```python
from build123d import *

# Parameters (mm, degrees)
SKETCH1_R           = 1.5
SKETCH1_R_2         = 4.25
SKETCH1_R_3         = 5
SKETCH1_R_4         = 1
BOSS_EXTRUDE2_DEPTH = 5
SKETCH2_W           = 0.5
SKETCH2_H           = 37
BOSS_EXTRUDE3_DEPTH = 5
CUT_EXTRUDE1_DEPTH  = 10
BOSS_EXTRUDE4_DEPTH = 5
SKETCH5_R           = 1.6
CUT_EXTRUDE2_DEPTH  = 10
BOSS_EXTRUDE5_DEPTH = 5
SKETCH7_R           = 1
BOSS_EXTRUDE6_DEPTH = 5
SKETCH8_W           = 5
SKETCH8_H           = 37
CUT_EXTRUDE3_DEPTH  = 33


with BuildPart() as part:
    # Sketch1 → Boss-Extrude2 (new body)
    with BuildSketch(Plane.XY):
        with BuildLine():
            Line((45.25091594, -25.207708346), (50.00091594, -20.457708346))
            Line((50.00091594, -20.457708346), (50.00091594, 24.688738263))
            Line((50.00091594, 24.688738263), (45.147362549, 29.542291654))
            Line((45.147362549, 29.542291654), (26.35446933, 29.542291654))
            Line((26.35446933, 29.542291654), (21.25091594, 24.438738263))
            Line((21.25091594, 24.438738263), (21.25091594, 18.042291654))
            Line((21.25091594, 18.042291654), (20.408095363, 18.042291654))
            Line((20.408095363, 18.042291654), (16.70086026, 18.042291654))
            ThreePointArc((16.70086026, 18.042291654), (12.892426636, 17.542145454), (9.3422674, 16.075624987))
            ThreePointArc((9.3422674, 16.075624987), (2.182128173, 13.100539865), (-5.49908406, 12.043324729))
            Line((-5.49908406, 12.043324729), (-5.49908406, 12.039085999))
            ThreePointArc((-5.49908406, 12.039085999), (-15.49908406, 2.292291654), (-5.49908406, -7.454502691))
            Line((-5.49908406, -7.454502691), (-5.49908406, -7.458741422))
            ThreePointArc((-5.49908406, -7.458741422), (2.182128173, -8.515956557), (9.3422674, -11.491041679))
            ThreePointArc((9.3422674, -11.491041679), (12.892426636, -12.957562146), (16.70086026, -13.457708346))
            Line((16.70086026, -13.457708346), (20.408095363, -13.457708346))
            Line((20.408095363, -13.457708346), (21.25091594, -13.457708346))
            Line((21.25091594, -13.457708346), (21.25091594, -20.207708346))
            Line((21.25091594, -20.207708346), (26.25091594, -25.207708346))
            Line((26.25091594, -25.207708346), (45.25091594, -25.207708346))
        make_face()
        with Locations((46.75091594, -7.707708346)):
            Circle(SKETCH1_R, mode=Mode.SUBTRACT)
        with Locations((46.75091594, 12.292291654)):
            Circle(SKETCH1_R, mode=Mode.SUBTRACT)
        with Locations((33.50091594, 14.792291654)):
            Circle(SKETCH1_R_2, mode=Mode.SUBTRACT)
        with Locations((33.50091594, -10.207708346)):
            Circle(SKETCH1_R_2, mode=Mode.SUBTRACT)
        with Locations((19.25091594, 12.292291654)):
            Circle(SKETCH1_R, mode=Mode.SUBTRACT)
        with Locations((19.25091594, -7.707708346)):
            Circle(SKETCH1_R, mode=Mode.SUBTRACT)
        with Locations((-5.74908406, 2.292291654)):
            Circle(SKETCH1_R_3, mode=Mode.SUBTRACT)
        with Locations((1.25091594, 2.354746229)):
            Circle(SKETCH1_R_4, mode=Mode.SUBTRACT)
        with Locations((-5.686629485, -4.707708346)):
            Circle(SKETCH1_R_4, mode=Mode.SUBTRACT)
        with Locations((-12.74908406, 2.229837079)):
            Circle(SKETCH1_R_4, mode=Mode.SUBTRACT)
        with Locations((-5.811538636, 9.292291654)):
            Circle(SKETCH1_R_4, mode=Mode.SUBTRACT)
    extrude(amount=BOSS_EXTRUDE2_DEPTH)

    # Sketch2 → Boss-Extrude3 (add)
    with BuildSketch(Plane(origin=(0, 0, 0), x_dir=(-1, 0, 0), z_dir=(0, 0, -1))):
        Polygon((-26.25091594, -25.207708346), (-21.50091594, -25.207708346), (-21.50091594, -20.457708346), align=None)
        Polygon((-45.25091594, -25.207708346), (-45.50091594, -25.207708346), (-45.50091594, -24.957708346), align=None)
        Polygon((-45.50091594, 29.188738263), (-45.50091594, 29.792291654), (-21.50091594, 29.792291654), (-21.50091594, 24.688738263), (-26.35446933, 29.542291654), (-45.147362549, 29.542291654), align=None)
        with Locations((-50.25091594, 2.292291654)):
            Rectangle(SKETCH2_W, SKETCH2_H)
    extrude(amount=-BOSS_EXTRUDE3_DEPTH)

    # Sketch3 → Cut-Extrude1 (cut)
    with BuildSketch(Plane(origin=(0, 0, 0), x_dir=(-1, 0, 0), z_dir=(0, 0, -1))):
        Polygon((-50.00091594, -16.207708346), (-45.50091594, -16.207708346), (-45.50091594, -25.207708346), (-50.00091594, -20.457708346), align=None)
        Polygon((-50.50091594, 20.792291654), (-45.50091594, 20.792291654), (-45.50091594, 29.188738263), (-50.00091594, 24.688738263), align=None)
        Polygon((-21.50091594, -16.207708346), (-21.50091594, -20.457708346), (-21.25091594, -20.207708346), (-21.25091594, -16.207708346), align=None)
        Polygon((-21.50091594, 20.792291654), (-21.25091594, 20.792291654), (-21.25091594, 24.438738263), (-21.50091594, 24.688738263), align=None)
    extrude(amount=-CUT_EXTRUDE1_DEPTH, mode=Mode.SUBTRACT)

    # Sketch4 → Boss-Extrude4 (add)
    with BuildSketch(Plane(origin=(0, 0, 0), x_dir=(-1, 0, 0), z_dir=(0, 0, -1))):
        with BuildLine():
            Line((-21.25091594, 20.792291654), (-16.50091594, 20.792291654))
            Line((-16.50091594, 20.792291654), (-16.50091594, 18.040936414))
            ThreePointArc((-16.50091594, 18.040936414), (-16.600885803, 18.04195284), (-16.70086026, 18.042291654))
            Line((-16.70086026, 18.042291654), (-21.25091594, 18.042291654))
            Line((-21.25091594, 18.042291654), (-21.25091594, 20.792291654))
        make_face()
        with BuildLine():
            Line((-16.50091594, -13.456353106), (-16.50091594, -16.207708346))
            Line((-16.50091594, -16.207708346), (-21.25091594, -16.207708346))
            Line((-21.25091594, -16.207708346), (-21.25091594, -13.457708346))
            Line((-21.25091594, -13.457708346), (-16.70086026, -13.457708346))
            ThreePointArc((-16.70086026, -13.457708346), (-16.600885803, -13.457369532), (-16.50091594, -13.456353106))
        make_face()
    extrude(amount=-BOSS_EXTRUDE4_DEPTH)

    # Sketch5 → Cut-Extrude2 (cut)
    with BuildSketch(Plane.XY.offset(5)):
        with Locations((20.50091594, -7.707708346)):
            Circle(SKETCH5_R)
        with Locations((20.50091594, 12.292291654)):
            Circle(SKETCH5_R)
    extrude(amount=-CUT_EXTRUDE2_DEPTH, mode=Mode.SUBTRACT)

    # Sketch6 → Boss-Extrude5 (add)
    with BuildSketch(Plane.XY.offset(5)):
        with BuildLine():
            ThreePointArc((19.75191594, -6.293848735), (18.90091594, -7.707708346), (19.75191594, -9.121567957))
            ThreePointArc((19.75191594, -9.121567957), (17.75091594, -7.707708346), (19.75191594, -6.293848735))
        make_face()
        with BuildLine():
            ThreePointArc((19.75191594, 13.706151265), (18.90091594, 12.292291654), (19.75191594, 10.878432043))
            ThreePointArc((19.75191594, 10.878432043), (17.75091594, 12.292291654), (19.75191594, 13.706151265))
        make_face()
    extrude(amount=-BOSS_EXTRUDE5_DEPTH)

    # Sketch7 → Boss-Extrude6 (add)
    with BuildSketch(Plane(origin=(0, 0, 0), x_dir=(-1, 0, 0), z_dir=(0, 0, -1))):
        with Locations((-1.25091594, 2.354746229)):
            Circle(SKETCH7_R)
        with Locations((12.74908406, 2.229837079)):
            Circle(SKETCH7_R)
    extrude(amount=-BOSS_EXTRUDE6_DEPTH)

    # Sketch8 → Cut-Extrude3 (cut, through all)
    with BuildSketch(Plane.ZY.offset(-16.50091594)):
        with Locations((2.5, 2.292291654)):
            Rectangle(SKETCH8_W, SKETCH8_H)
    extrude(amount=CUT_EXTRUDE3_DEPTH, mode=Mode.SUBTRACT)


solid = part.part
```
The model under review builds one solid part; all positions refer to its coordinate system, in mm. A direction names the side the tool comes from. Round coordinates to 2 decimals unless told otherwise and drop trailing zeros. Order: outer loops, then holes, each group sorted by start corner. A loop starts at its lowest first (then second) coordinate and runs counter-clockwise, first axis right, second up.
(1) Take a section at C-C, the plane y = 22.5. State the section outline as (x, z) points.
Working result:
outline: (21.5, 0) - (45.5, 0) - (45.5, 5) - (21.5, 5) - close
(2) For P1, Ø2.5, axis at y = -21, z = 3, coming from the +X side; P2, Ø3, axis at x = 20.5, y = -7.71, coming from the +Z side; P3, Ø4, axis at x = 46.75, y = -7.71, coming from the -Z side; P4, Ø1.5, axis at y = 24.5, z = 1.5, coming from the -X side, all flat-tipped, find the tip position at first contact; note any pin that passes through.
Working result:
P1: stops at x = 45.5
P2: passes through
P3: stops at z = 0
P4: stops at x = 21.5
(3) Mouldability with a two-part tool opening along Y and no side actions: class faces 5 (the face through (21.501, -21, 2)), 6 (the face through (19, 20.792, 2)), 7 (the face through (30.4, 17.7, 2.5)) as released by +Y, released by -Y, zero draft, split by the parting line, or undercut.
Working result:
face 5: zero draft
face 6: released by +Y
face 7: undercut
(4) Take a section at B-B, the plane z = 4.1. State the section outline as (x, y) points, plus the area to 3 significant figures.
Working result:
outline: (16.5, -16.21) - (21.5, -16.21) - (21.5, -25.21) - (45.5, -25.21) - (45.5, -16.21) - (50.5, -16.21) - (50.5, 20.79) - (45.5, 20.79) - (45.5, 29.79) - (21.5, 29.79) - (21.5, 20.79) - (16.5, 20.79) - close; hole circle Ø3.2 at (20.5, -7.71); hole circle Ø3.2 at (20.5, 12.29); hole circle Ø8.5 at (33.5, -10.21); hole circle Ø8.5 at (33.5, 14.79); hole circle Ø3 at (46.75, -7.71); hole circle Ø3 at (46.75, 12.29)
area: 1,550 mm2
(5) Take a section at A-A, the plane y = -11. State the section outline as (x, z) points, plus the area to 3 significant figures.
Working result:
outline: (16.5, 0) - (29.33, 0) - (29.33, 5) - (16.5, 5) - close; (37.68, 0) - (50.5, 0) - (50.5, 5) - (37.68, 5) - close
area: 128 mm2
(6) Wall thickness on L1, parallel to Y at x = 33.5, z = 4.3; L2, parallel to X at y = -7, z = 1.45; L3, parallel to X at y = -9, z = 2.45: over which ranges is each line inside the solid? List them lowest first.
Working result:
L1: y = -25.21 to -14.46, -5.96 to 10.54, 19.04 to 29.79
L2: x = 16.5 to 19.07, 21.94 to 30.71, 36.29 to 45.43, 48.07 to 50.5
L3: x = 16.5 to 19.56, 21.44 to 29.43, 37.58 to 45.99, 47.51 to 50.5
(7) Tool access review of faces 1 (the face through (19, -16.208, 2)), 2 (the face through (21.501, 25, 2)), 3 (the face through (45.501, -21, 2)), 4 (the face through (45.501, 25, 2)): name each direction out of +Z, -Z, +X, -X, +Y, -Y from which nothing blocks a thin tool from reaching the whole face with its end or side.
Working result:
face 1: +Z, -Z, -X, -Y
face 2: +Z, -Z, -X, +Y
face 3: +Z, -Z, +X, -Y
face 4: +Z, -Z, +X, +Y
